from build123d import *

# Parameters (mm, degrees)
SKETCH1_W           = 52
SKETCH1_H           = 20
SKETCH1_R           = 2.1
BOSS_EXTRUDE1_DEPTH = 4
SKETCH2_W           = 52
SKETCH2_H           = 4
BOSS_EXTRUDE2_DEPTH = 48
CUT_EXTRUDE1_REACH  = 22
SKETCH3_R           = 2.1
BOSS_EXTRUDE3_DEPTH = 16
CUT_EXTRUDE3_DEPTH  = 53


with BuildPart() as part:
    # Sketch1 → Boss-Extrude1 (new body)
    with BuildSketch(Plane(origin=(0, 0, 0), x_dir=(1, 0, 0), z_dir=(0, 1, 0))):
        with Locations((26, 10)):
            Rectangle(SKETCH1_W, SKETCH1_H)
        with Locations((43.9, 10)):
            Circle(SKETCH1_R, mode=Mode.SUBTRACT)
        with Locations((8.1, 10)):
            Circle(SKETCH1_R, mode=Mode.SUBTRACT)
    extrude(amount=BOSS_EXTRUDE1_DEPTH)

    # Sketch2 → Boss-Extrude2 (add)
    with BuildSketch(Plane.XZ):
        with Locations((26, -2)):
            Rectangle(SKETCH2_W, SKETCH2_H)
    extrude(amount=BOSS_EXTRUDE2_DEPTH)

    # Sketch3 → Cut-Extrude1 (cut, up to next)
    with BuildSketch(Plane.XY, mode=Mode.PRIVATE) as cut_extrude1_sk1:
        with Locations((26, -41)):
            Circle(SKETCH3_R)
    cut_extrude1_tool1 = extrude(cut_extrude1_sk1.sketch, amount=-CUT_EXTRUDE1_REACH, mode=Mode.PRIVATE) & part.part
    add(cut_extrude1_tool1.solids().sort_by_distance((26, -41, 0))[0], mode=Mode.SUBTRACT)
    # Sketch3 → Cut-Extrude1 (cut, up to next)
    with BuildSketch(Plane.XY, mode=Mode.PRIVATE) as cut_extrude1_sk2:
        Polygon((52, 0), (34.25, -48), (52, -48), align=None)
    cut_extrude1_tool2 = extrude(cut_extrude1_sk2.sketch, amount=-CUT_EXTRUDE1_REACH, mode=Mode.PRIVATE) & part.part
    add(cut_extrude1_tool2.solids().sort_by_distance((46.083333, -32, 0))[0], mode=Mode.SUBTRACT)
    # Sketch3 → Cut-Extrude1 (cut, up to next)
    with BuildSketch(Plane.XY, mode=Mode.PRIVATE) as cut_extrude1_sk3:
        Polygon((0, -48), (0, 0), (17.75, -48), align=None)
    cut_extrude1_tool3 = extrude(cut_extrude1_sk3.sketch, amount=-CUT_EXTRUDE1_REACH, mode=Mode.PRIVATE) & part.part
    add(cut_extrude1_tool3.solids().sort_by_distance((5.916667, -32, 0))[0], mode=Mode.SUBTRACT)

    # Sketch5 → Boss-Extrude3 (add)
    with BuildSketch(Plane(origin=(0, 0, -4), x_dir=(-1, 0, 0), z_dir=(0, 0, -1))):
        Polygon((-34.25, -48), (-38.012268219, 0), (-34, 0), (-30.237731781, -48), align=None)
        Polygon((-13.987731781, 0), (-18, 0), (-21.762268219, -48), (-17.75, -48), align=None)
    extrude(amount=BOSS_EXTRUDE3_DEPTH)

    # Sketch6 → Cut-Extrude3 (cut, through all)
    with BuildSketch(Plane.ZY):
        Polygon((-20, 0), (-4, -48), (-20, -48), align=None)
    extrude(amount=-CUT_EXTRUDE3_DEPTH, mode=Mode.SUBTRACT)


solid = part.part
Build history of the part. All positions in model axes, mm. A direction names the side the tool comes from. Coordinates: 2 decimals unless noted, no trailing zeros. Order: outer loops, then holes, each group sorted by start corner. A loop starts at its lowest first (then second) coordinate and runs counter-clockwise, first axis right, second up. Notation, with made-up numbers: (16, 77.25) - (53, 77.25) arc R11 ccw to (53, 89.25) - close; hole circle Ø9 at (-3.75, -31). An arc over 180 degrees is marked (long way). Put each result on its own line as item: value.
1. Saw through at D-D (y = -22). Write the cut outline in (x, z).
Answer sheet:
outline: (8.14, -4) - (15.71, -4) - (15.71, -12.67) - (19.72, -12.67) - (19.72, -4) - (32.28, -4) - (32.28, -12.67) - (36.29, -12.67) - (36.29, -4) - (43.86, -4) - (43.86, 0) - (8.14, 0) - close
2. Saw through at C-C (z = -1.75). Write the cut outline in (x, y).
Answer sheet:
outline: (0, 0) - (17.75, -48) - (34.25, -48) - (52, 0) - (52, 4) - (0, 4) - close; hole circle Ø4.2 at (26, -41)
3. Drop flat-ended pins along their axis: P1, Ø11, axis at x = 44.5, z = -11.5, coming from the -Y side; P2, Ø19.5, axis at x = 6, y = -33, coming from the -Z side; P3, Ø2, axis at y = -4, z = -5.5, coming from the +X side; P4, Ø4, axis at x = 8.1, z = -10, coming from the -Y side. Give the stop position or say it passes through.
Answer sheet:
P1: stops at y = 0
P2: stops at z = -4
P3: stops at x = 37.78
P4: passes through
4. Saw through at B-B (z = -8.75). Write the cut outline in (x, y), and give its area (3 significant figures).
Answer sheet:
outline: (0, 0) - (6.41, 0) - (6.41, 4) - (0, 4) - close; (9.79, 0) - (13.99, 0) - (16.63, -33.75) - (20.65, -33.75) - (18, 0) - (34, 0) - (31.35, -33.75) - (35.37, -33.75) - (38.01, 0) - (42.21, 0) - (42.21, 4) - (9.79, 4) - close; (45.59, 0) - (52, 0) - (52, 4) - (45.59, 4) - close
area: 452 mm^2
5. Pull direction X, two halves, no side cores. Call faces 6 (the face through (42.352, 1.972, -11.419)), 7 (the face through (0, 2, -10)), 8 (the face through (52, 2, -10)): pulls with the +X half, pulls with the -X half, needs draft (parallel to the pull), parting line crosses it, or undercut.
Answer sheet:
face 6: undercut
face 7: pulls with the -X half
face 8: pulls with the +X half
6. Saw through at A-A (x = 26). Write the cut outline in (y, z), and give its area (3 significant figures).
Answer sheet:
outline: (-48, -4) - (-43.1, -4) - (-43.1, 0) - (-48, 0) - close; (-38.9, -4) - (0, -4) - (0, -20) - (4, -20) - (4, 0) - (-38.9, 0) - close
area: 255 mm^2
7. Probe line 1 along Z through (x, y) = (43.9, 2.4); line 2 along Z through (x, y) = (5.5, -1); line 3 along X through (y, z) = (-9, -5.5). List the from-to ranges inside material, lowest first. Write a range as [from, to].
Answer sheet:
line 1: z = [-20, -12.1], [-7.9, 0]
line 2: z = [-4, 0]
line 3: x = [14.69, 18.71], [33.29, 37.31]
8. Tool access for faces 1 (the face through (41, -18, -4)), 2 (the face through (32.563, -18.331, -10.11)), 3 (the face through (26, 4, -10)), 4 (the face through (34, -24, -12)), 5 (the face through (7, 0, -12)): list every direction of +Z, -Z, +X, -X, +Y, -Y with a clear straight run to the whole face (end or side of a thin tool).
Answer sheet:
face 1: -Z, +X, -Y
face 2: -Z
face 3: +Z, -Z, +X, -X, +Y
face 4: -Z, +X, -X, -Y
face 5: -Z, -X, -Y
